Build history of the part. All positions in model axes, mm. A direction names the side the tool comes from. Give positions to 0.01 mm unless a question says otherwise; leave off trailing zeros. Loops run counter-clockwise (first coordinate to the right, second up) from the corner with the lowest first, then second, coordinate; pieces in that order, holes last. Notation, with made-up numbers: (37, 49) -> (42, 49) arc R18 cw to (42, 55) -> close; hole circle Ø10 at (39, 44). An arc over 180 degrees is marked (long way). One line per question, with ' | ' between items. Start each with the question number.
(1) Slice it at C-C, the plane z = -8. Write the cut outline in (x, y), then the cut area to 3 significant figures.
(2) Slice it at B-B, the plane x = 8.25. Write the cut outline in (y, z).
(3) Slice it at A-A, the plane z = 0. Give the number of separate pieces and of enclosed holes in the cut face, then the cut area to 3 significant figures.
(4) Flat gauge pins, fed straight in: pin 1 Ø8 at (x, z) = (-7.5, 7) entering from -Y; pin 2 Ø10 at (y, z) = (7, 5.5) entering from -X; pin 3 Ø4.5 at (x, z) = (-7.5, 1) entering from +Y; pin 4 Ø1.5 at (y, z) = (15, -3) entering from -X. Where does each tip first touch, or does it go through?
(5) Drill centre lines: L1, parallel to Z at x = 0, y = 1.3; L2, parallel to Z at x = 0, y = 2.5. Where is each one in solid material? Low to high. Write a range as from..to.
(6) Mould opens along X. For faces 4 (the face through (10.6, 1.94, -3.34)), 5 (the face through (-0.563, 1.158, -6.918)), 6 (the face through (-3, 3.937, 2)), 7 (the face through (0.16, 1.16, 6.79)) say: pulls with the +X half, pulls with the -X half, needs draft (parallel to the pull), parting line crosses it, or undercut.
(7) 3-axis set-ups, long thin cutter, end or side, ignore diameter. For faces 1 (the face through (-0.633, 23.915, 2.852)), 2 (the face through (1, 2.35, -9)), 3 (the face through (0, 32.385, 0)): which of +Z, -Z, +X, -X, +Y, -Y reach the whole face in a straight line?
```python
from build123d import *

# Parameters (mm, degrees)
SKETCH1_R                       = 11.1125
BOSS_EXTRUDE1_DEPTH             = 3.937
BOSS_EXTRUDE2_START             = -3.937
SKETCH2_R                       = 3.175
BOSS_EXTRUDE2_DEPTH             = 32.385
F_2_CLEARANCE_HOLE1_D           = 2.4384
SKETCH5_R                       = 1.984375
CUT_EXTRUDE1_DEPTH              = 1.5875
F_3_32_0_09375_DIAMETER_HOLE1_D = 2.38125
CUT_EXTRUDE2_START              = -8.85825
SKETCH9_R                       = 3.175
SKETCH9_R_2                     = 2.921
CUT_EXTRUDE2_DEPTH              = 0.7874


with BuildPart() as part:
    # Sketch1 → Boss-Extrude1 (new body)
    with BuildSketch(Plane(origin=(0, 0, 0), x_dir=(1, 0, 0), z_dir=(0, 1, 0))):
        Circle(SKETCH1_R)
    extrude(amount=BOSS_EXTRUDE1_DEPTH)

    # Sketch2 → Boss-Extrude2 (add)
    with BuildSketch(Plane(origin=(0, 3.937, 0), x_dir=(1, 0, 0), z_dir=(0, 1, 0)).offset(BOSS_EXTRUDE2_START)):
        Circle(SKETCH2_R)
    extrude(amount=BOSS_EXTRUDE2_DEPTH)

    # #2 Clearance Hole1 (through all)
    with Locations(Plane(origin=(0, 3.937, 0), x_dir=(1, 0, 0), z_dir=(0, 1, 0))):
        with Locations((0, -8), (0, 8), (-8, 0), (8, 0)):
            Hole(F_2_CLEARANCE_HOLE1_D / 2)

    # Sketch5 → Cut-Extrude1 (cut)
    with BuildSketch(Plane(origin=(0, 3.937, 0), x_dir=(1, 0, 0), z_dir=(0, 1, 0))):
        with Locations((0, -8)):
            Circle(SKETCH5_R)
        with Locations((8, 0)):
            Circle(SKETCH5_R)
        with Locations((0, 8)):
            Circle(SKETCH5_R)
        with Locations((-8, 0)):
            Circle(SKETCH5_R)
    extrude(amount=-CUT_EXTRUDE1_DEPTH, mode=Mode.SUBTRACT)

    # 3/32 (0.09375) Diameter Hole1 (through all)
    with Locations(Plane.XY.offset(3.175)):
        with Locations((0, 14.144625)):
            Hole(F_3_32_0_09375_DIAMETER_HOLE1_D / 2)

    # Sketch9 → Cut-Extrude2 (cut)
    with BuildSketch(Plane(origin=(0, 32.385, 0), x_dir=(1, 0, 0), z_dir=(0, 1, 0)).offset(CUT_EXTRUDE2_START)):
        Circle(SKETCH9_R)
        Circle(SKETCH9_R_2, mode=Mode.SUBTRACT)
    extrude(amount=CUT_EXTRUDE2_DEPTH, mode=Mode.SUBTRACT)


solid = part.part
```
Final values:
1) outline: (-7.71, 0) -> (-1.22, 0) -> (-1.22, 2.35) -> (-1.98, 2.35) -> (-1.98, 3.94) -> (-7.71, 3.94) -> close; (1.22, 0) -> (7.71, 0) -> (7.71, 3.94) -> (1.98, 3.94) -> (1.98, 2.35) -> (1.22, 2.35) -> close | area: 48.7 mm2
2) outline: (0, -7.44) -> (3.94, -7.44) -> (3.94, -1.97) -> (2.35, -1.97) -> (2.35, -1.19) -> (0, -1.19) -> close; (0, 1.19) -> (2.35, 1.19) -> (2.35, 1.97) -> (3.94, 1.97) -> (3.94, 7.44) -> (0, 7.44) -> close
3) separate pieces: 3 | enclosed holes: 1 | area: 239 mm2
4) pin 1: y = 0 | pin 2: x = -11 | pin 3: y = 3.94 | pin 4: x = -2.24
5) L1: -11.11..-9.22, -6.78..6.78, 9.22..11.11 | L2: -11.11..-9.98, -6.02..6.02, 9.98..11.11
6) face 4: parting line crosses it | face 5: undercut | face 6: needs draft | face 7: undercut
7) face 1: none | face 2: +Y | face 3: +Z, -Z, +X, -X, +Y
